from build123d import *

# Parameters (mm, degrees)
SKETCH_1_W      = 108
SKETCH_1_H      = 60.88
SKETCH_1_R      = 1.6
EXTRUDE_1_DEPTH = 1.6
SKETCH_2_W      = 94.6
SKETCH_2_H      = 60.88
EXTRUDE_2_DEPTH = 4.85
SKETCH_3_W      = 3
SKETCH_3_H      = 35.56
EXTRUDE_3_DEPTH = 8.34


with BuildPart() as part:
    # 草图1 → 凸台-拉伸1 (new body)
    with BuildSketch(Plane(origin=(0, 0, 0), x_dir=(1, 0, 0), z_dir=(0, 1, 0))):
        with Locations((54, 30.44)):
            Rectangle(SKETCH_1_W, SKETCH_1_H)
        with Locations(Location((3, 57.88, 0), (0, 0, 270))):
            Circle(SKETCH_1_R, mode=Mode.SUBTRACT)
        with Locations(Location((3, 3, 0), (0, 0, 270))):
            Circle(SKETCH_1_R, mode=Mode.SUBTRACT)
        with Locations(Location((105, 3, 0), (0, 0, 90))):
            Circle(SKETCH_1_R, mode=Mode.SUBTRACT)
        with Locations(Location((105, 57.88, 0), (0, 0, 90))):
            Circle(SKETCH_1_R, mode=Mode.SUBTRACT)
    extrude(amount=EXTRUDE_1_DEPTH)

    # 草图2 → 凸台-拉伸2 (add)
    with BuildSketch(Plane(origin=(0, 1.6, 0), x_dir=(1, 0, 0), z_dir=(0, 1, 0))):
        with Locations((54, 30.44)):
            Rectangle(SKETCH_2_W, SKETCH_2_H)
    extrude(amount=EXTRUDE_2_DEPTH)

    # 草图3 → 凸台-拉伸3 (add)
    with BuildSketch(Plane.XZ):
        with Locations((1.5, -30.44)):
            Rectangle(SKETCH_3_W, SKETCH_3_H)
    extrude(amount=EXTRUDE_3_DEPTH)


solid = part.part
Check sheet for the modelled part. Datum: model origin and axes. Units: mm. A direction names the side the tool comes from. Give positions to 0.01 mm unless a question says otherwise; leave off trailing zeros. Loops run counter-clockwise (first coordinate to the right, second up) from the corner with the lowest first, then second, coordinate; pieces in that order, holes last. Notation, with made-up numbers: M 21,24.5 L 46,24.5 A8 ccw 46,35.5 Z; hole C -33,59.25 d3. An arc over 180 degrees is marked long. Answer as a JSON object with one key per item and string values. Group by question number.
Q1. Material ranges on line 1 along Z through (x, y) = (105, 0.5); line 2 along X through (y, z) = (1.25, -3); line 3 along Y through (x, z) = (28, -58), recorded low to high. Write a range as [from, to].
Q2. Release check for a two-part mould opening along Z. For faces 1 (the cylindrical face through (103.414, 0.789, -2.792)), 2 (the flat face through (1, -8.34, -30)), 3 (the flat face through (53, 3, -60.88)) record: released by +Z, released by -Z, zero draft, split by the parting line, or undercut.
Q3. Cross-section at A-A on z = -3. Record the cut outline in (x, y).
Q4. Go/stop test with flat-tipped pins: P1, Ø2, axis at x = 103.5, z = -33, coming from the +Y side; P2, Ø2.5, axis at y = 4.5, z = -26.5, coming from the +X side; P3, Ø2.5, axis at x = 1, y = -2, coming from the -Z side. Record where each tip stops, or that it passes through.
Q5. Access from +Z, -Z, +X, -X, +Y, -Y to the whole of each face (thin tool, end or side, straight path). Record for faces 4 (the flat face through (101.3, 4, -30)), 5 (the flat face through (1, -4, -48.22)), 6 (the flat face through (6.7, 4, -30)), 7 (the flat face through (3, -4, -31)).
Q6. Cross-section at D-D on y = -6.5. Record the cut outline in (x, z), then the cut area to 3 significant figures.
Q7. Cross-section at C-C on z = -32.5. Record the cut outline in (x, y), then the cut area to 3 significant figures.
Q8. Cross-section at B-B on x = 105. Record the cut outline in (y, z).
Evaluation:
{
 "1": {"line 1": "z = [-60.88, -59.48], [-56.28, -4.6], [-1.4, 0]", "line 2": "x = [0, 1.4], [4.6, 103.4], [106.6, 108]", "line 3": "y = [0, 6.45]"},
 "2": {"face 1": "undercut", "face 2": "zero draft", "face 3": "released by -Z"},
 "3": {"outline": "M 0,0 L 1.4,0 L 1.4,1.6 L 0,1.6 Z; M 4.6,0 L 103.4,0 L 103.4,1.6 L 101.3,1.6 L 101.3,6.45 L 6.7,6.45 L 6.7,1.6 L 4.6,1.6 Z; M 106.6,0 L 108,0 L 108,1.6 L 106.6,1.6 Z"},
 "4": {"P1": "stops at y = 1.6", "P2": "stops at x = 101.3", "P3": "stops at z = -48.22"},
 "5": {"face 4": "+Z, -Z, +X, +Y", "face 5": "-Z, +X, -X, -Y", "face 6": "+Z, -Z, -X, +Y", "face 7": "+Z, -Z, +X, -Y"},
 "6": {"outline": "M 0,-48.22 L 3,-48.22 L 3,-12.66 L 0,-12.66 Z", "area": "107 mm2"},
 "7": {"outline": "M 0,-8.34 L 3,-8.34 L 3,0 L 108,0 L 108,1.6 L 101.3,1.6 L 101.3,6.45 L 6.7,6.45 L 6.7,1.6 L 0,1.6 Z", "area": "657 mm2"},
 "8": {"outline": "M 0,-60.88 L 1.6,-60.88 L 1.6,-59.48 L 0,-59.48 Z; M 0,-56.28 L 1.6,-56.28 L 1.6,-4.6 L 0,-4.6 Z; M 0,-1.4 L 1.6,-1.4 L 1.6,0 L 0,0 Z"}
}
